Part model, mm, in its own coordinate system. A direction names the side the tool comes from. Give positions to 0.01 mm unless a question says otherwise; leave off trailing zeros. Write each loop counter-clockwise with the first axis right and the second up, starting at its lowest first coordinate (ties: lowest second). Pieces come first, ordered by that corner, then holes.
```python
from build123d import *

# Parameters (mm, degrees)
SKETCH1_W           = 8
SKETCH1_H           = 70
BOSS_EXTRUDE1_DEPTH = 15
SKETCH2_W           = 10
SKETCH2_H           = 3
BOSS_EXTRUDE2_DEPTH = 12
SKETCH3_R           = 2.6
CUT_EXTRUDE1_DEPTH  = 12
FILLET1_R           = 5
SCALE1_SCALE        = 0.7


with BuildPart() as part:
    # Sketch1 → Boss-Extrude1 (new body)
    with BuildSketch(Plane(origin=(0, 0, 0), x_dir=(0, 1, 0), z_dir=(0, 0, 1))):
        Rectangle(SKETCH1_W, SKETCH1_H)
    extrude(amount=-BOSS_EXTRUDE1_DEPTH)

    # Sketch2 → Boss-Extrude2 (add)
    with BuildSketch(Plane.XZ.offset(4)):
        with Locations((0, -3.8)):
            Rectangle(SKETCH2_W, SKETCH2_H)
        with Locations((0, -11.3)):
            Rectangle(SKETCH2_W, SKETCH2_H)
    extrude(amount=BOSS_EXTRUDE2_DEPTH)

    # Sketch3 → Cut-Extrude1 (cut)
    with BuildSketch(Plane.XY.offset(-2.3)):
        with Locations((0, -10)):
            Circle(SKETCH3_R)
    extrude(amount=-CUT_EXTRUDE1_DEPTH, mode=Mode.SUBTRACT)

    # Fillet1
    fillet1_edges = [part.edges().sort_by_distance(p)[0] for p in [
        (-5, -16, -11.3),
        (5, -16, -11.3),
        (5, -16, -3.8),
        (-5, -16, -3.8),
    ]]
    fillet(fillet1_edges, radius=FILLET1_R - 0.0001)  # a hair under: the kernel refuses the full size


with BuildPart() as part_1:
    # Scale1: scaled about (0, -0.556396742, -7.502958038)
    add(part.part.scale(SCALE1_SCALE).moved(Location((0, -0.166919023, -2.250887411))))


solid = part_1.part
```
1) Wall check: L1, parallel to Y at x = 0, z = -5.3; L2, parallel to Z at x = 0, y = -4.75; L3, parallel to Y at x = -22, z = -6.75. Give the ranges that are in metal, low to high.
Answers follow:
L1: y = -11.37 to -8.99, -5.35 to 2.63
L2: z = -11.21 to -9.11, -5.96 to -3.86
L3: y = -2.97 to 2.63
2) Saw through at C-C, the plane x = 10. Write the cut outline in (y, z).
Answers follow:
outline: (-2.97, -12.75) - (2.63, -12.75) - (2.63, -2.25) - (-2.97, -2.25) - close
3) Saw through at D-D, the plane z = -7.75. Write the cut outline in (x, y), then the cut area to 3 significant figures.
Answers follow:
outline: (-24.5, -2.97) - (24.5, -2.97) - (24.5, 2.63) - (-24.5, 2.63) - close
area: 274 mm2
4) Saw through at A-A, the plane y = -4.5. Write the cut outline in (x, z), then the cut area to 3 significant figures.
Answers follow:
outline: (-3.5, -11.21) - (3.5, -11.21) - (3.5, -9.11) - (-3.5, -9.11) - close; (-3.5, -5.96) - (3.5, -5.96) - (3.5, -3.86) - (-3.5, -3.86) - close
area: 29.4 mm2
5) 3-axis set-ups, long thin cutter, end or side, ignore diameter. For faces 4 (the face through (3.5, -5, -5)), 5 (the face through (0, -5, -11.211)), 6 (the face through (0, -5, -3.861)): which of +Z, -Z, +X, -X, +Y, -Y reach the whole face in a straight line?
Answers follow:
face 4: +Z, -Z, +X, -Y
face 5: -Z, +X, -X, -Y
face 6: +Z, +X, -X, -Y
6) Pin check, flat tips, straight feed: pin 1 Ø1.1 at (y, z) = (-6.5, -10) entering from -X; pin 2 Ø1.1 at (y, z) = (-4.5, -10.5) entering from +X; pin 3 Ø2 at (x, z) = (-5.5, -7.5) entering from -Y. Stop position of each tip, or through.
Answers follow:
pin 1: stops at x = -3.5
pin 2: stops at x = 3.5
pin 3: stops at y = -2.97
7) Two-plate mould, pull along X, no slides. Class faces 1 (the face through (-0.237, -5.362, -4.896)), 2 (the face through (3.5, -5, -10)), 3 (the face through (0, -2.967, -7)): +X half, -X half, draft (parallel to the pull), parting line (faces both ways), or undercut.
Answers follow:
face 1: undercut
face 2: +X half
face 3: draft
